Geometry check sheet. Reference: the model listing, model coordinates, mm. A direction names the side the tool comes from. Coordinates: 2 decimals unless noted, no trailing zeros. Write each loop counter-clockwise with the first axis right and the second up, starting at its lowest first coordinate (ties: lowest second). Pieces come first, ordered by that corner, then holes. Notation, with made-up numbers: (25, -28) -> (30, -28) arc R15 ccw to (30, -11) -> close; hole circle Ø4 at (82.5, 60.5). An arc over 180 degrees is marked (long way). Put each result on its own line as item: value. Start each with the question number.
from build123d import *

# Parameters (mm, degrees)
PAD_DEPTH                          = 3
SKETCH001_W                        = 6.6
SKETCH001_H                        = 6.6
POCKET_DEPTH                       = 2
SKETCH002_W                        = 1.1
SKETCH002_H                        = 0.8
POCKET001_DEPTH                    = 86.372938
SKETCH002_LINEARPATTERN_2_W        = 1.1
SKETCH002_LINEARPATTERN_2_H        = 0.8
POCKET001_LINEARPATTERN_2_DEPTH    = 86.372938
SKETCH001_LINEARPATTERN_2_W        = 6.6
SKETCH001_LINEARPATTERN_2_H        = 6.6
POCKET_LINEARPATTERN_2_DEPTH       = 2
LINEARPATTERN001_COUNT             = 2
LINEARPATTERN001_PITCH             = 9.8
SKETCH001_LINEARPATTERN002_2_W     = 6.6
SKETCH001_LINEARPATTERN002_2_H     = 6.6
POCKET_LINEARPATTERN002_2_DEPTH    = 2
SKETCH002_LINEARPATTERN002_2_W     = 1.1
SKETCH002_LINEARPATTERN002_2_H     = 0.8
POCKET001_LINEARPATTERN002_2_DEPTH = 86.372938
LINEARPATTERN003_COUNT             = 2
LINEARPATTERN003_PITCH             = 9.8
FILLET_R                           = 2


with BuildPart() as part:
    # Sketch → Pad (new body)
    with BuildSketch(Plane.XY):
        Polygon((-4.9, 4.9), (-4.9, 14.7), (4.9, 14.7), (4.9, 4.9), (14.7, 4.9), (14.7, -4.9), (4.9, -4.9), (4.9, -14.7), (-4.9, -14.7), (-4.9, -4.9), (-14.7, -4.9), (-14.7, 4.9), align=None)
    extrude(amount=PAD_DEPTH)

    # Sketch001 (on Face14 of Pad) → Pocket (cut)
    with BuildSketch(Plane.XY.offset(3)):
        Rectangle(SKETCH001_W, SKETCH001_H)
    pocket = extrude(amount=-POCKET_DEPTH, mode=Mode.SUBTRACT)

    # Sketch002 (on Face5 of Pocket) → Pocket001 (cut, through all)
    with BuildSketch(Plane.XY.offset(3)):
        with Locations((-2.25, 3.5)):
            Rectangle(SKETCH002_W, SKETCH002_H)
        with Locations((2.25, 3.5)):
            Rectangle(SKETCH002_W, SKETCH002_H)
        with Locations((2.25, -3.5)):
            Rectangle(SKETCH002_W, SKETCH002_H)
        with Locations((-2.25, -3.5)):
            Rectangle(SKETCH002_W, SKETCH002_H)
    pocket001 = extrude(amount=-POCKET001_DEPTH, mode=Mode.SUBTRACT)

    # Sketch002 LinearPattern 2 → Pocket001 LinearPattern 2 (cut, through all)
    with BuildSketch(Plane(origin=(9.8, 0, 3), x_dir=(1, 0, 0), z_dir=(0, 0, 1))):
        with Locations((-2.25, 3.5)):
            Rectangle(SKETCH002_LINEARPATTERN_2_W, SKETCH002_LINEARPATTERN_2_H)
        with Locations((2.25, 3.5)):
            Rectangle(SKETCH002_LINEARPATTERN_2_W, SKETCH002_LINEARPATTERN_2_H)
        with Locations((2.25, -3.5)):
            Rectangle(SKETCH002_LINEARPATTERN_2_W, SKETCH002_LINEARPATTERN_2_H)
        with Locations((-2.25, -3.5)):
            Rectangle(SKETCH002_LINEARPATTERN_2_W, SKETCH002_LINEARPATTERN_2_H)
    pocket001_linearpattern_2 = extrude(amount=-POCKET001_LINEARPATTERN_2_DEPTH, mode=Mode.SUBTRACT)

    # Sketch001 LinearPattern 2 → Pocket LinearPattern 2 (cut)
    with BuildSketch(Plane(origin=(9.8, 0, 3), x_dir=(1, 0, 0), z_dir=(0, 0, 1))):
        Rectangle(SKETCH001_LINEARPATTERN_2_W, SKETCH001_LINEARPATTERN_2_H)
    pocket_linearpattern_2 = extrude(amount=-POCKET_LINEARPATTERN_2_DEPTH, mode=Mode.SUBTRACT)

    # LinearPattern001: Pocket001, Pocket, Pocket001 LinearPattern 2, Pocket LinearPattern 2 ×2
    with Locations(*[(-i * LINEARPATTERN001_PITCH, 0, 0) for i in range(1, LINEARPATTERN001_COUNT)]):
        add(pocket001, mode=Mode.SUBTRACT)
        add(pocket, mode=Mode.SUBTRACT)
        add(pocket001_linearpattern_2, mode=Mode.SUBTRACT)
        add(pocket_linearpattern_2, mode=Mode.SUBTRACT)

    # Sketch001 LinearPattern002 2 → Pocket LinearPattern002 2 (cut)
    with BuildSketch(Plane(origin=(0, 9.8, 3), x_dir=(1, 0, 0), z_dir=(0, 0, 1))):
        Rectangle(SKETCH001_LINEARPATTERN002_2_W, SKETCH001_LINEARPATTERN002_2_H)
    pocket_linearpattern002_2 = extrude(amount=-POCKET_LINEARPATTERN002_2_DEPTH, mode=Mode.SUBTRACT)

    # Sketch002 LinearPattern002 2 → Pocket001 LinearPattern002 2 (cut, through all)
    with BuildSketch(Plane(origin=(0, 9.8, 3), x_dir=(1, 0, 0), z_dir=(0, 0, 1))):
        with Locations((-2.25, 3.5)):
            Rectangle(SKETCH002_LINEARPATTERN002_2_W, SKETCH002_LINEARPATTERN002_2_H)
        with Locations((2.25, 3.5)):
            Rectangle(SKETCH002_LINEARPATTERN002_2_W, SKETCH002_LINEARPATTERN002_2_H)
        with Locations((2.25, -3.5)):
            Rectangle(SKETCH002_LINEARPATTERN002_2_W, SKETCH002_LINEARPATTERN002_2_H)
        with Locations((-2.25, -3.5)):
            Rectangle(SKETCH002_LINEARPATTERN002_2_W, SKETCH002_LINEARPATTERN002_2_H)
    pocket001_linearpattern002_2 = extrude(amount=-POCKET001_LINEARPATTERN002_2_DEPTH, mode=Mode.SUBTRACT)

    # LinearPattern003: Pocket, Pocket001, Pocket LinearPattern002 2, Pocket001 LinearPattern002 2 ×2
    with Locations(*[(0, -i * LINEARPATTERN003_PITCH, 0) for i in range(1, LINEARPATTERN003_COUNT)]):
        add(pocket, mode=Mode.SUBTRACT)
        add(pocket001, mode=Mode.SUBTRACT)
        add(pocket_linearpattern002_2, mode=Mode.SUBTRACT)
        add(pocket001_linearpattern002_2, mode=Mode.SUBTRACT)

    # Fillet
    fillet_edges = [part.edges().sort_by_distance(p)[0] for p in [
        (-4.9, -4.9, 1.5),
        (4.9, -4.9, 1.5),
        (4.9, 4.9, 1.5),
        (-4.9, 4.9, 1.5),
    ]]
    fillet(fillet_edges, radius=FILLET_R)


solid = part.part
Item 1: Section check B-B, the plane y = 10.25. Enter the section's corners in (x, z).
Item 2: Scan lines: line 1 along X through (y, z) = (-1.5, 2.6); line 2 along Y through (x, z) = (10.5, 1.25). Record each from-to range of solid material in increasing order. Write a range as [from, to].
Item 3: Section check A-A, the plane x = 12.25. Enter the section's corners in (y, z), and give its area (3 significant figures).
Item 4: Section check C-C, the plane z = 0.5. Give the number of separate pieces and of enclosed holes in the cut face, and give its area (3 significant figures).
Item 5: Mould release check, pull along Y, two halves, no side actions. Record for faces 3 (the flat face through (0, 14.7, 1)), 4 (the flat face through (-11.5, -3.6, 1.5)): released by +Y, released by -Y, zero draft, split by the parting line, or undercut.
Item 6: Go/stop test with flat-tipped pins: P1, Ø0.9, axis at x = 7.5, z = 2, coming from the -Y side; P2, Ø0.9, axis at x = -7.5, z = 1, coming from the +Y side; P3, Ø1, axis at y = -10.5, z = 0.5, coming from the +X side. Record where each tip stops, or that it passes through.
Item 7: Access from +Z, -Z, +X, -X, +Y, -Y to the whole of each face (thin tool, end or side, straight path). Record for faces 1 (the flat face through (0, 13.1, 2)), 2 (the flat face through (7.5, 3.9, 1.5)).
From the geometry:
1. outline: (-4.9, 0) -> (4.9, 0) -> (4.9, 3) -> (3.3, 3) -> (3.3, 1) -> (-3.3, 1) -> (-3.3, 3) -> (-4.9, 3) -> close
2. line 1: [-14.7, -13.1], [-6.5, -3.3], [3.3, 6.5], [13.1, 14.7]
2. line 2: [-4.9, -3.3], [3.3, 4.9]
3. outline: (-4.9, 0) -> (-3.9, 0) -> (-3.9, 3) -> (-4.9, 3) -> close; (-3.1, 0) -> (3.1, 0) -> (3.1, 1) -> (-3.1, 1) -> close; (3.9, 0) -> (4.9, 0) -> (4.9, 3) -> (3.9, 3) -> close
3. area: 12.2 mm²
4. separate pieces: 1
4. enclosed holes: 20
4. area: 466 mm²
5. face 3: released by +Y
5. face 4: undercut
6. P1: y = -4.9
6. P2: y = 4.9
6. P3: x = 4.9
7. face 1: +Z
7. face 2: +Z, -Z
